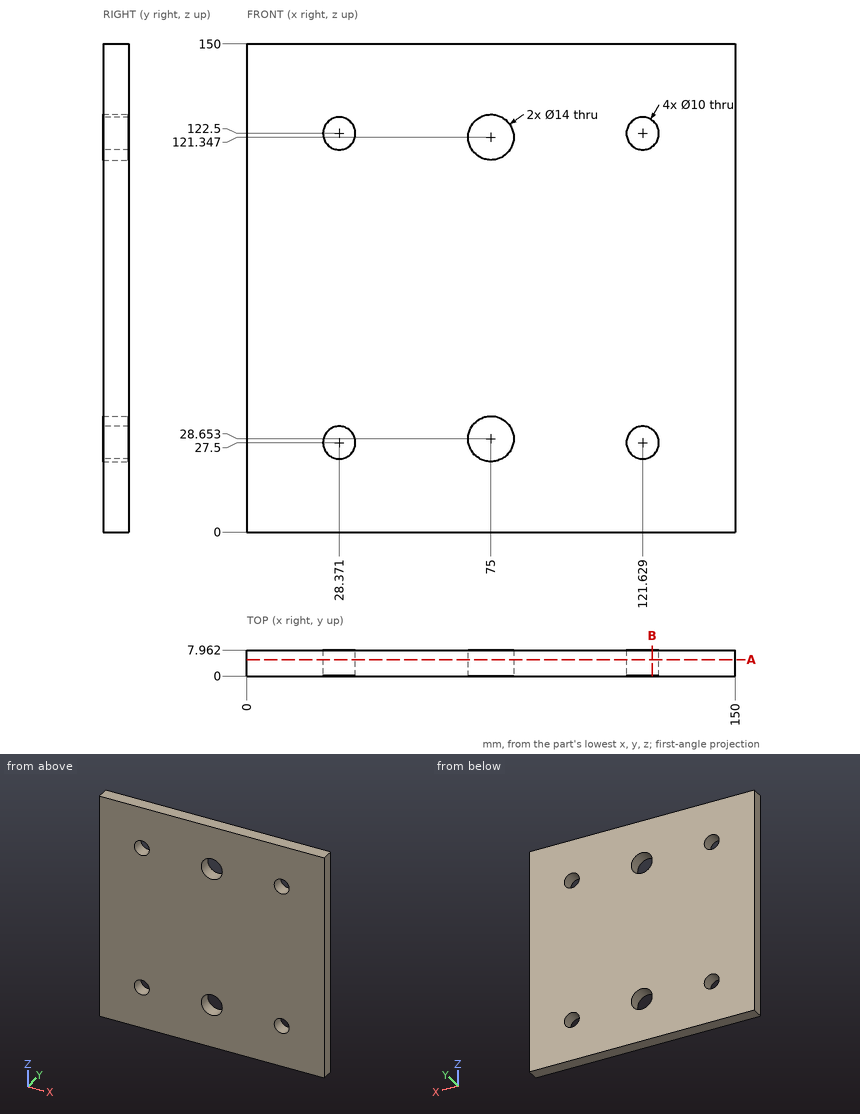
Design review of the part shown in the three views and the two pictorial views. Dimensions are in mm from the part's minimum x, y and z. Coordinates: 2 decimals unless noted, no trailing zeros. Write each loop counter-clockwise with the first axis right and the second up, starting at its lowest first coordinate (ties: lowest second). Pieces come first, ordered by that corner, then holes.
(1) Wall thickness on probe 1 along Z at (x, y) = (29, 1.5); probe 2 along Z at (x, y) = (120.5, 4.25); probe 3 along X at (y, z) = (6.25, 125.5) (1 decimal): over which ranges is each line inside the solid? List them lowest first.
(2) Add section B-B on x = 124.5. Give the boundary of the cut face in (y, z), then the cut area to 3 significant figures.
(3) Add section A-A on y = 5. Give the boundary of the cut face in (x, z).
Answer sheet:
1. probe 1: z = 0 to 22.54, 32.46 to 117.54, 127.46 to 150
1. probe 2: z = 0 to 22.63, 32.37 to 117.63, 127.37 to 150
1. probe 3: x = 0 to 24.4, 32.4 to 69.4, 80.6 to 117.6, 125.6 to 150
2. outline: (0, 0) - (7.96, 0) - (7.96, 23.41) - (0, 23.41) - close; (0, 31.59) - (7.96, 31.59) - (7.96, 118.41) - (0, 118.41) - close; (0, 126.59) - (7.96, 126.59) - (7.96, 150) - (0, 150) - close
2. area: 1,060 mm2
3. outline: (0, 0) - (150, 0) - (150, 150) - (0, 150) - close; hole circle Ø10 at (28.37, 27.5); hole circle Ø10 at (28.37, 122.5); hole circle Ø14 at (75, 28.65); hole circle Ø14 at (75, 121.35); hole circle Ø10 at (121.63, 27.5); hole circle Ø10 at (121.63, 122.5)
